Input: part model. Units: mm. Frame: model coordinates. Give positions to 0.01 mm unless a question says otherwise; leave off trailing zeros. Answer as a JSON object with one key per item and string values.
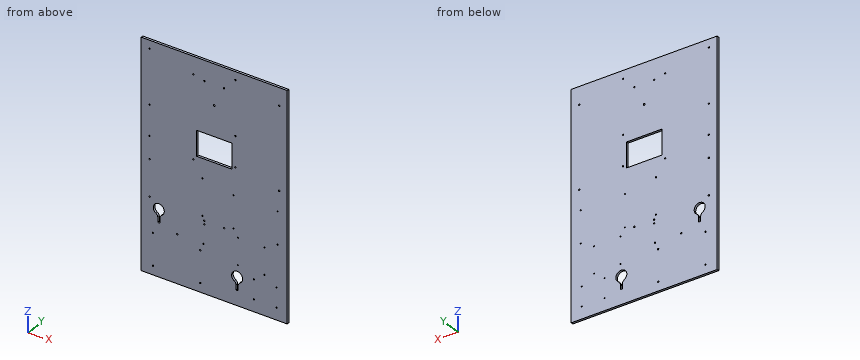
```python
from build123d import *

# Parameters (mm, degrees)
SKETCH1_R           = 1.778
SKETCH1_R_2         = 1.397
BOSS_EXTRUDE1_DEPTH = 5.6388
SKETCH5_R           = 2.39395
CUT_EXTRUDE1_DEPTH  = 6.6388
SKETCH6_R           = 1.778
CUT_EXTRUDE2_DEPTH  = 6.6388
SKETCH7_W           = 90.6
SKETCH7_H           = 63.5
CUT_EXTRUDE3_DEPTH  = 6.6388


with BuildPart() as part:
    # Sketch1 → Boss-Extrude1 (new body)
    with BuildSketch(Plane(origin=(0, 0, 0), x_dir=(1, 0, 0), z_dir=(0, 1, 0))):
        Polygon((-836.762809235, 790.243336478), (-836.762809235, 232.943336478), (-836.762809235, 226.593336478), (-466.762809235, 226.593336478), (-466.762809235, 232.943336478), (-466.762809235, 790.243336478), (-466.762809235, 796.593336478), (-836.762809235, 796.593336478), align=None)
        with Locations((-807.062809235, 774.087336478)):
            Circle(SKETCH1_R, mode=Mode.SUBTRACT)
        with Locations((-807.062809235, 694.087336478)):
            Circle(SKETCH1_R, mode=Mode.SUBTRACT)
        with Locations((-687.062809235, 694.087336478)):
            Circle(SKETCH1_R, mode=Mode.SUBTRACT)
        with Locations((-687.062809235, 774.087336478)):
            Circle(SKETCH1_R, mode=Mode.SUBTRACT)
        with Locations((-551.437809235, 766.168335733)):
            Circle(SKETCH1_R_2, mode=Mode.SUBTRACT)
        with Locations((-551.437809235, 717.168335733)):
            Circle(SKETCH1_R_2, mode=Mode.SUBTRACT)
        with Locations((-493.437809235, 717.168335733)):
            Circle(SKETCH1_R_2, mode=Mode.SUBTRACT)
        with Locations((-493.437809235, 766.168335733)):
            Circle(SKETCH1_R_2, mode=Mode.SUBTRACT)
        with Locations((-591.737808414, 696.968336156)):
            Circle(SKETCH1_R_2, mode=Mode.SUBTRACT)
        with Locations((-591.737808414, 629.968336156)):
            Circle(SKETCH1_R_2, mode=Mode.SUBTRACT)
        with Locations((-524.737808414, 629.968336156)):
            Circle(SKETCH1_R_2, mode=Mode.SUBTRACT)
        with Locations((-524.737808414, 696.968336156)):
            Circle(SKETCH1_R_2, mode=Mode.SUBTRACT)
        with Locations((-815.553809235, 608.213336478)):
            Circle(SKETCH1_R, mode=Mode.SUBTRACT)
        with Locations((-681.441809235, 608.213336478)):
            Circle(SKETCH1_R, mode=Mode.SUBTRACT)
        with Locations((-681.441809235, 516.773336478)):
            Circle(SKETCH1_R, mode=Mode.SUBTRACT)
        with Locations((-815.553809235, 516.773336478)):
            Circle(SKETCH1_R, mode=Mode.SUBTRACT)
        with Locations((-602.652809235, 611.403336478)):
            Circle(SKETCH1_R_2, mode=Mode.SUBTRACT)
        with Locations((-602.652809235, 530.123336478)):
            Circle(SKETCH1_R_2, mode=Mode.SUBTRACT)
        with Locations((-490.892809235, 611.403336478)):
            Circle(SKETCH1_R_2, mode=Mode.SUBTRACT)
        with Locations((-490.892809235, 530.123336478)):
            Circle(SKETCH1_R_2, mode=Mode.SUBTRACT)
        with Locations((-487.082809235, 478.673336478)):
            Circle(SKETCH1_R, mode=Mode.SUBTRACT)
        with Locations((-598.080809235, 460.258336478)):
            Circle(SKETCH1_R, mode=Mode.SUBTRACT)
        with Locations((-598.080809235, 384.058336478)):
            Circle(SKETCH1_R, mode=Mode.SUBTRACT)
        with Locations((-487.082809235, 271.091836478)):
            Circle(SKETCH1_R, mode=Mode.SUBTRACT)
        with Locations((-598.080809235, 247.152336478)):
            Circle(SKETCH1_R, mode=Mode.SUBTRACT)
        with Locations((-704.682809235, 271.091836478)):
            Circle(SKETCH1_R, mode=Mode.SUBTRACT)
        with Locations((-815.680809235, 247.152336478)):
            Circle(SKETCH1_R, mode=Mode.SUBTRACT)
        with Locations((-815.680809235, 384.058336478)):
            Circle(SKETCH1_R, mode=Mode.SUBTRACT)
        with Locations((-815.680809235, 460.258336478)):
            Circle(SKETCH1_R, mode=Mode.SUBTRACT)
        with Locations((-704.682809235, 478.673336478)):
            Circle(SKETCH1_R, mode=Mode.SUBTRACT)
        with Locations((-678.940809235, 675.739236478)):
            Circle(SKETCH1_R, mode=Mode.SUBTRACT)
        with Locations((-745.539609235, 675.739236478)):
            Circle(SKETCH1_R, mode=Mode.SUBTRACT)
        with Locations((-676.790809235, 627.495236478)):
            Circle(SKETCH1_R, mode=Mode.SUBTRACT)
    extrude(amount=BOSS_EXTRUDE1_DEPTH)

    # Sketch5 → Cut-Extrude1 (cut, through all)
    with BuildSketch(Plane.XZ):
        with Locations((-651.762809235, -328.193336478)):
            Circle(SKETCH5_R)
        with BuildLine():
            Line((-794.852809235, -664.280486837), (-794.852809235, -651.921486174))
            ThreePointArc((-794.852809235, -651.921486174), (-796.125971484, -647.038628109), (-799.62126981, -643.399104156))
            ThreePointArc((-799.62126981, -643.399104156), (-792.312809235, -617.523336478), (-785.004348659, -643.399104156))
            ThreePointArc((-785.004348659, -643.399104156), (-788.499646985, -647.038628109), (-789.772809235, -651.921486174))
            Line((-789.772809235, -651.921486174), (-789.772809235, -664.280486837))
            Line((-789.772809235, -664.280486837), (-794.852809235, -664.280486837))
        make_face()
        with BuildLine():
            Line((-596.302809235, -759.530486837), (-596.302809235, -747.171486174))
            ThreePointArc((-596.302809235, -747.171486174), (-597.575971484, -742.288628109), (-601.07126981, -738.649104156))
            ThreePointArc((-601.07126981, -738.649104156), (-593.762809235, -712.773336478), (-586.454348659, -738.649104156))
            ThreePointArc((-586.454348659, -738.649104156), (-589.949646985, -742.288628109), (-591.222809235, -747.171486174))
            Line((-591.222809235, -747.171486174), (-591.222809235, -759.530486837))
            Line((-591.222809235, -759.530486837), (-596.302809235, -759.530486837))
        make_face()
    extrude(amount=-CUT_EXTRUDE1_DEPTH, mode=Mode.SUBTRACT)

    # Sketch6 → Cut-Extrude2 (cut, through all)
    with BuildSketch(Plane(origin=(0, 5.6388, 0), x_dir=(1, 0, 0), z_dir=(0, 1, 0))):
        with Locations((-676.762809235, 277.393336478)):
            Circle(SKETCH6_R)
        with Locations((-626.762809235, 277.393336478)):
            Circle(SKETCH6_R)
        with Locations((-676.762809235, 618.593336478)):
            Circle(SKETCH6_R)
        with Locations((-626.762809235, 618.593336478)):
            Circle(SKETCH6_R)
    extrude(amount=-CUT_EXTRUDE2_DEPTH, mode=Mode.SUBTRACT)

    # Sketch7 → Cut-Extrude3 (cut, through all)
    with BuildSketch(Plane(origin=(0, 5.6388, 0), x_dir=(1, 0, 0), z_dir=(0, 1, 0))):
        with Locations((-651.762809235, 436.143336478)):
            Rectangle(SKETCH7_W, SKETCH7_H)
    extrude(amount=-CUT_EXTRUDE3_DEPTH, mode=Mode.SUBTRACT)


solid = part.part
```
Q1. Section A-A, the plane y = 1.2. Give the number of separate pieces and of enclosed holes in the cut face, then the cut area to 3 significant figures.
Evaluation:
{"separate pieces": "1", "enclosed holes": "41", "area": "203,000 mm2"}
Q2. Ray query, line 1 along Z through (x, y) = (-815.5, 1.2); line 2 along Z through (x, y) = (-493, 3.9); line 3 along Z through (x, y) = (-674, 1.95). Return the intervals inside material, ascending.
Evaluation:
{"line 1": "z = -796.59 to -609.99, -606.44 to -518.55, -515 to -462.03, -458.49 to -385.83, -382.29 to -248.92, -245.38 to -226.59", "line 2": "z = -796.59 to -767.49, -764.84 to -718.49, -715.84 to -226.59", "line 3": "z = -796.59 to -467.89, -404.39 to -226.59"}
Q3. Pin query (flat end, axial travel): pin 1 (4.5 mm diameter, centred on x = -490.89, z = -530.12, fed in from +Y). Return the tip coordinate at first contact, or that it passes through.
Evaluation:
{"pin 1": "stops at y = 5.64"}
